Can you work these out from the model? Positions are in its coordinate system, mm. A direction names the side the tool comes from. Give positions to 0.01 mm unless a question says otherwise; leave off trailing zeros. Order: outer loops, then holes, each group sorted by start corner. A loop starts at its lowest first (then second) coordinate and runs counter-clockwise, first axis right, second up. Notation, with made-up numbers: (-36.75, 72) -> (12.25, 72) arc R23 ccw to (12.25, 102) -> close; hole circle Ø8 at (41.25, -5). An arc over 180 degrees is marked (long way). Answer as a JSON object with one key per item and string values.
Autodesk Inventor part; units mm, degrees
ref_plane "YZ Plane" through (0, 0, 0) normal (1, 0, 0) x (0, 1, 0)
ref_plane "XZ Plane" through (0, 0, 0) normal (0, 1, 0) x (-1, 0, 0)
ref_plane "XY Plane" through (0, 0, 0) normal (0, 0, 1) x (1, 0, 0)
sketch "Sketch1" plane through (0, 0, 0) normal (0, 0, 1) x (1, 0, 0)
  arc A0 (-36.3497, -18.0713) -> (-15.9827, -32.4309) centre (-25.5909, -24.4351) ccw
  arc A1 (35.8842, -10.6617) -> (38.9651, 7.8249) centre (35.8842, -1.1617) ccw
  arc A2 (-1.287, 21.6247) -> (-16.0996, 16.1641) centre (-5.3408, 9.8003) ccw
  arc A3 (12.4467, -10.6617) -> (-4.4637, -18.5891) centre (12.4467, -32.6617) ccw
  line L0 (-15.9827, -32.4309) -> (-4.4637, -18.5891)
  line L1 (12.4467, -10.6617) -> (35.8842, -10.6617)
  line L2 (38.9651, 7.8249) -> (-1.287, 21.6247)
  line L3 (-16.0996, 16.1641) -> (-36.3497, -18.0713)
  dimension "d0" = 12.5
  dimension "d1" = 9.5
  dimension "d2" = 12.5
  dimension "d3" = 22
extrude "Extrusion1" add sketch "Sketch1" along normal mid plane 6.5
sketch "Sketch2" plane through (0, 0, 3.25) normal (0, 0, 1) x (1, 0, 0)
  arc A0 (-36.3497, -18.0713) -> (-15.9827, -32.4309) centre (-25.5909, -24.4351) ccw
  arc A1 (-1.287, 21.6247) -> (-16.0996, 16.1641) centre (-5.3408, 9.8003) ccw
  arc A2 (35.8842, -10.6617) -> (38.9651, 7.8249) centre (35.8842, -1.1617) ccw
  line L0 (-36.3497, -18.0713) -> (-16.0996, 16.1641)
  line L1 (-4.4637, -18.5891) -> (-15.9827, -32.4309)
  arc A3 (12.4467, -10.6617) -> (-4.4637, -18.5891) centre (12.4467, -32.6617) ccw
  line L2 (35.8842, -10.6617) -> (12.4467, -10.6617)
  line L3 (-1.287, 21.6247) -> (38.9651, 7.8249)
hole "Hole1" at (-25.5909, -24.4351, 3.25) direction (0, 0, -1) diameter 10 end through all
sketch "Sketch3" plane through (0, 0, 3.25) normal (0, 0, 1) x (1, 0, 0)
  arc A0 (-1.287, 21.6247) -> (-16.0996, 16.1641) centre (-5.3408, 9.8003) ccw
hole "Hole2" at (-5.3408, 9.8003, 3.25) direction (0, 0, -1) diameter 15 end through all
sketch "Sketch4" plane through (0, 0, 3.25) normal (0, 0, 1) x (1, 0, 0)
  arc A0 (35.8842, -10.6617) -> (38.9651, 7.8249) centre (35.8842, -1.1617) ccw
hole "Hole3" at (35.8842, -1.1617, 3.25) direction (0, 0, -1) diameter 10 end through all
fillet "Fillet1" radius 1 16 edges at (18.8391, 14.7248, 3.25) (45.2549, -2.7234, 3.25) (24.1654, -10.6617, 3.25) (3.1086, -12.7419, 3.25) (-10.2232, -25.51, 3.25) (-32.7937, -34.6512, 3.25) (-26.2246, -0.9536, 3.25) (-9.6644, 21.5287, 3.25) (18.8391, 14.7248, -3.25) (-9.6644, 21.5287, -3.25) (-26.2246, -0.9536, -3.25) (-32.7937, -34.6512, -3.25) (-10.2232, -25.51, -3.25) (3.1086, -12.7419, -3.25) (24.1654, -10.6617, -3.25) (45.2549, -2.7234, -3.25)
properties part number "Bracket - Optimization - Copy" material "Aluminum 6061"
1. Will these pins go through, and if not, where does the flat tip stop? pin 1 Ø2 at (x, y) = (-4.5, 14.5) entering from +Z; pin 2 Ø3 at (x, z) = (-2, 0) entering from +Y; pin 3 Ø2 at (y, z) = (-14.5, 0) entering from +X.
Worked answers:
{"pin 1": "through", "pin 2": "y = 22.16", "pin 3": "x = 1.64"}
2. For faces 4 (the face through (24, -10.662, 0)), 5 (the face through (-9.776, 21.487, -0.031)), which set-ups out of +Z, -Z, +X, -X, +Y, -Y let a thin tool reach every point of the face, with its end or its side?
Worked answers:
{"face 4": "+Z, -Z, +X, -Y", "face 5": "+Z, -Z, +Y"}
3. If we mould it in two halves opening along Y, with no side actions, what happens to faces 1 (the face through (40.32, -3.47, -0.05)), 2 (the face through (-10.36, -25.23, -2.95)), 3 (the face through (-26.08, -0.71, -0.03))? For each: +Y half, -Y half, draft (parallel to the pull), parting line (faces both ways), or undercut.
Worked answers:
{"face 1": "undercut", "face 2": "-Y half", "face 3": "+Y half"}
4. Please list where these lines run through material, in increasing order: L1, parallel to X at y = -21, z = -3; L2, parallel to X at y = -26, z = -2.75; L3, parallel to Y at x = -26, z = 2.75.
Worked answers:
{"L1": "-37.26 to -29.22, -21.96 to -6.91", "L2": "-37.86 to -30.34, -20.84 to -10.81", "L3": "-36.79 to -29.42, -19.45 to -0.84"}
5. If we section it at A-A on z = -1: Please give me the cut outline in (x, y), then the cut area to 3 significant figures.
Worked answers:
{"outline": "(-36.35, -18.07) arc R12.5 ccw to (-15.98, -32.43) -> (-4.46, -18.59) arc R22 cw to (12.45, -10.66) -> (35.88, -10.66) arc R9.5 ccw to (38.97, 7.82) -> (-1.29, 21.62) arc R12.5 ccw to (-16.1, 16.16) -> close; hole circle Ø10 at (-25.59, -24.44); hole circle Ø15 at (-5.34, 9.8); hole circle Ø10 at (35.88, -1.16)", "area": "2,170 mm²"}
